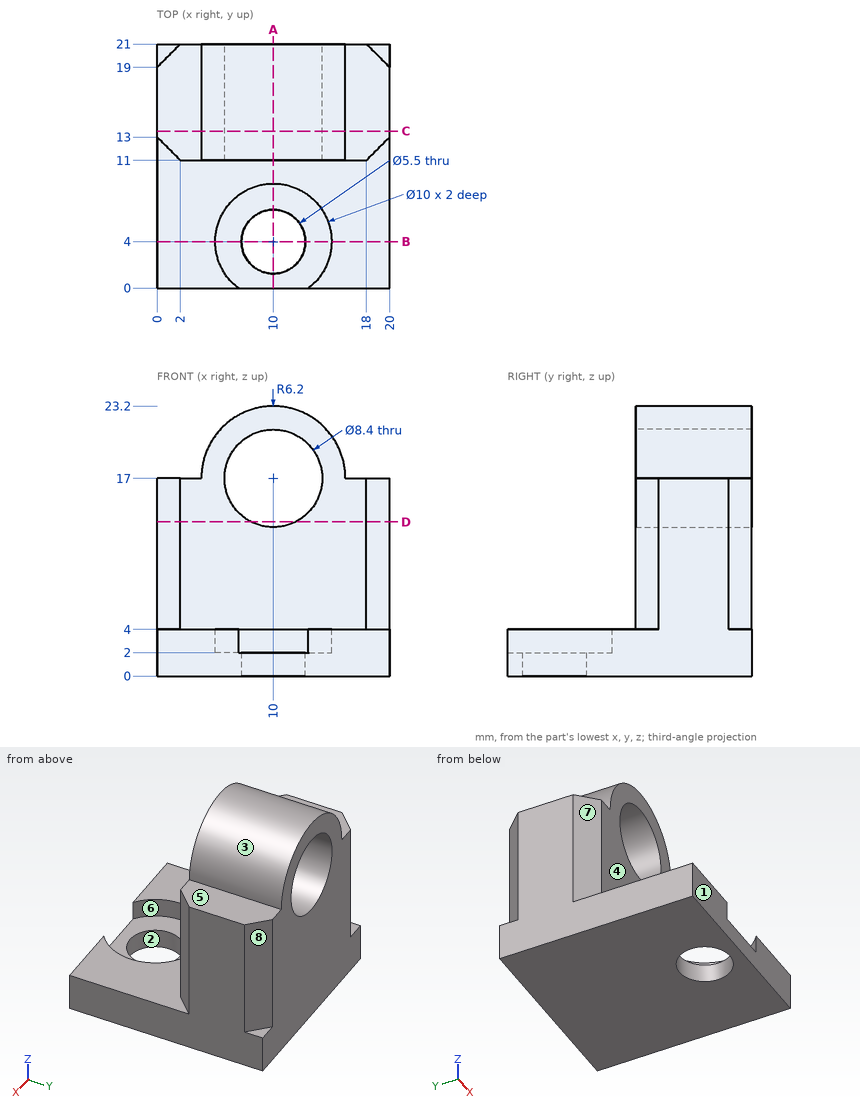
The figure shows three views and two pictorial views of one solid part (mm, origin at its lowest corner). Answer the questions. A direction names the side the tool comes from. Give positions to 0.01 mm unless a question says otherwise; leave off trailing zeros. Write each loop counter-clockwise with the first axis right and the second up, starting at its lowest first coordinate (ties: lowest second). Pieces come first, ordered by that corner, then holes. Notation, with made-up numbers: (-37.5, -26.75) -> (-26.5, -26.75) arc R10 cw to (-26.5, -20.75) -> close; hole circle Ø8 at (77, -0.75). An arc over 180 degrees is marked (long way). Answer as a JSON object with one key per item and string values.
1) Straight lines are drawn through the part: probe 1 along X at (y, z) = (4, 2.75); probe 2 along Y at (x, z) = (10, 1.65); probe 3 along X at (y, z) = (4, 1.25). For each, find the intervals that lie inside material, in ascending order. Write a range as from..to.
Findings below:
{"probe 1": "x = 0..5, 15..20", "probe 2": "y = 0..1.25, 6.75..21", "probe 3": "x = 0..7.25, 12.75..20"}
2) Section A-A on x = 10 is taken. Write down the section's boundary in (y, z).
Findings below:
{"outline": "(0, 0) -> (1.25, 0) -> (1.25, 2) -> (0, 2) -> close; (6.75, 0) -> (21, 0) -> (21, 12.8) -> (11, 12.8) -> (11, 4) -> (9, 4) -> (9, 2) -> (6.75, 2) -> close; (11, 21.2) -> (21, 21.2) -> (21, 23.2) -> (11, 23.2) -> close"}
3) Section C-C on y = 13.5 is taken. Write down the section's boundary in (x, z).
Findings below:
{"outline": "(0, 0) -> (20, 0) -> (20, 17) -> (16.2, 17) arc R6.2 ccw to (3.8, 17) -> (0, 17) -> close; hole circle Ø8.4 at (10, 17)"}
4) For a pull along Y with two mould halves and no side action, classify the marked faces 1, 2 and 3 as pulls with the +Y half, pulls with the -Y half, needs draft (parallel to the pull), parting line crosses it, or undercut.
Findings below:
{"face 1": "pulls with the -Y half", "face 2": "undercut", "face 3": "needs draft"}
5) A tool of negligible diameter and unlimited length cuts with its end or side. For the marked faces 4, 5, 6, 7 and 8, from which of +Z, -Z, +X, -X, +Y, -Y can it reach the whole face along a straight path? Write none if from no direction.
Findings below:
{"face 4": "+Z, +X, -X, -Y", "face 5": "+Z, +X, +Y, -Y", "face 6": "+Z", "face 7": "+Z, -X, -Y", "face 8": "+Z, +X, +Y"}
6) Section B-B on y = 4 is taken. Write down the section's boundary in (x, z), then the cut area to 3 significant figures.
Findings below:
{"outline": "(0, 0) -> (7.25, 0) -> (7.25, 2) -> (5, 2) -> (5, 4) -> (0, 4) -> close; (12.75, 0) -> (20, 0) -> (20, 4) -> (15, 4) -> (15, 2) -> (12.75, 2) -> close", "area": "49.0 mm^2"}
7) Flat-ended cylindrical pins translate along their axes: pin 1 Ø6 at (x, y) = (9, 11.5) entering from -Z; pin 2 Ø4 at (x, y) = (5, 6) entering from +Z; pin 3 Ø4.5 at (x, y) = (10.5, 5) entering from +Z; pin 4 Ø1 at (x, y) = (19, 20.5) entering from +Z. Find the tip coordinate at first contact, or state that the pin passes through.
Findings below:
{"pin 1": "stops at z = 0", "pin 2": "stops at z = 4", "pin 3": "stops at z = 2", "pin 4": "stops at z = 17"}
8) Section D-D on z = 13.25 is taken. Write down the section's boundary in (x, y), then the cut area to 3 significant figures.
Findings below:
{"outline": "(0, 13) -> (2, 11) -> (8.11, 11) -> (8.11, 21) -> (2, 21) -> (0, 19) -> close; (11.89, 11) -> (18, 11) -> (20, 13) -> (20, 19) -> (18, 21) -> (11.89, 21) -> close", "area": "154 mm^2"}
